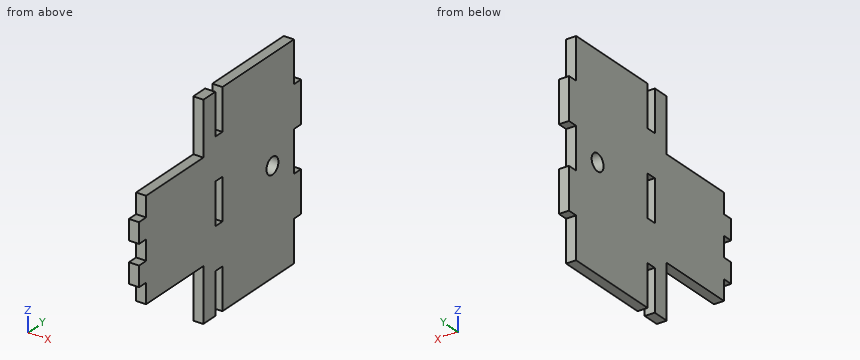
```python
from build123d import *

# Parameters (mm, degrees)
SKETCH1_R           = 2.5
SKETCH1_W           = 12.4
SKETCH1_H           = 3
BOSS_EXTRUDE3_DEPTH = 3


with BuildPart() as part:
    # Sketch1 → Boss-Extrude3 (new body)
    with BuildSketch(Plane(origin=(0, 0, 0), x_dir=(0, 0, -1), z_dir=(1, 0, 0))):
        Polygon((31, -2), (31, -7), (15, -7), (15, -31), (9, -31), (9, -34), (3, -34), (3, -31), (-3, -31), (-3, -34), (-9, -34), (-9, -31), (-15, -31), (-15, -7), (-31, -7), (-31, -2), (-18.6, -2), (-18.6, 1), (-31, 1), (-31, 31), (-18.6, 31), (-18.6, 34), (-6.2, 34), (-6.2, 31), (6.2, 31), (6.2, 34), (18.6, 34), (18.6, 31), (31, 31), (31, 1), (18.6, 1), (18.6, -2), align=None)
        with Locations((0, 22)):
            Circle(SKETCH1_R, mode=Mode.SUBTRACT)
        with Locations((0, -0.5)):
            Rectangle(SKETCH1_W, SKETCH1_H, mode=Mode.SUBTRACT)
    extrude(amount=BOSS_EXTRUDE3_DEPTH)


solid = part.part
```
Can you work these out from the model? Positions are in its coordinate system, mm. Give positions to 0.01 mm unless a question says otherwise; leave off trailing zeros. Write each loop counter-clockwise with the first axis right and the second up, starting at its lowest first coordinate (ties: lowest second). Pieces come first, ordered by that corner, then holes. Notation, with made-up numbers: (-14.75, 30) -> (3.25, 30) arc R29 cw to (3.25, 52) -> close; hole circle Ø5 at (68, 24). An arc over 180 degrees is marked (long way). Write item = value, one per line.
(1) Suppose I cut it at A-A on z = 0. Write out the boundary of the cut face in (x, y).
Worked out:
outline = (0, -31) -> (3, -31) -> (3, -2) -> (0, -2) -> close; (0, 1) -> (3, 1) -> (3, 19.5) -> (0, 19.5) -> close; (0, 24.5) -> (3, 24.5) -> (3, 31) -> (0, 31) -> close
(2) I need wall thicknesses on probe 1 along Y at (x, z) = (1.5, 0); probe 2 along Y at (x, z) = (1.05, 5.5); probe 3 along Y at (x, z) = (1.65, -1.5). Which ranges of each line are inside material? Lowest first, please. Write a range as from..to.
Worked out:
probe_1 = -31..-2, 1..19.5, 24.5..31
probe_2 = -34..-2, 1..31
probe_3 = -31..-2, 1..20, 24..31
(3) Suppose I cut it at B-B on y = 22. Write out the boundary of the cut face in (x, z).
Worked out:
outline = (0, -31) -> (3, -31) -> (3, -2.5) -> (0, -2.5) -> close; (0, 2.5) -> (3, 2.5) -> (3, 31) -> (0, 31) -> close
(4) I'm going to push flat-ended pins straight in: P1, Ø0.9, axis at x = 1.5, z = 11, coming from the -Y side; P2, Ø0.9, axis at x = 2, z = 3, coming from the +Y side; P3, Ø0.9, axis at x = 1.5, y = 33, coming from the +Z side. Where does each tip first touch, or does it pass through?
Worked out:
P1 = -31
P2 = 31
P3 = 18.6
(5) Suppose I cut it at D-D on z = 13.5. Write out the boundary of the cut face in (x, y).
Worked out:
outline = (0, -31) -> (3, -31) -> (3, 34) -> (0, 34) -> close
(6) Suppose I cut it at C-C on x = 1.2. Count the separate pieces of the cut face and the enclosed holes in it, then the cut area to 3 significant figures.
Worked out:
separate_pieces = 1
enclosed_holes = 2
area = 3,060 mm^2
